from build123d import *

# Parameters (mm, degrees)
F4_W = 133.35
F4_H = 38.1
F0_W = 133.35
F0_H = 66.675
F6_T = -2.54


with BuildPart() as f5:
    # F4 (on face) → F5 section 0
    with BuildSketch(Plane(origin=(0, -59.055, 59.055), x_dir=(1, 0, 0), z_dir=(0, 0.7071067812, -0.7071067812))):
        with Locations((60.325, 0.0451280605)):
            Rectangle(F4_W, F4_H)
    # F0 (on Top) → F5 section 1
    with BuildSketch(Plane.XY):
        with Locations((60.325, 26.9875)):
            Rectangle(F0_W, F0_H)
    loft()

    # F6
    f6_openings = [f5.faces().sort_by_distance(p)[0] for p in [
        (60.325, 26.9875, 0),
        (60.325, -59.08691, 59.02309),
    ]]
    offset(amount=F6_T, openings=f6_openings)


solid = f5.part
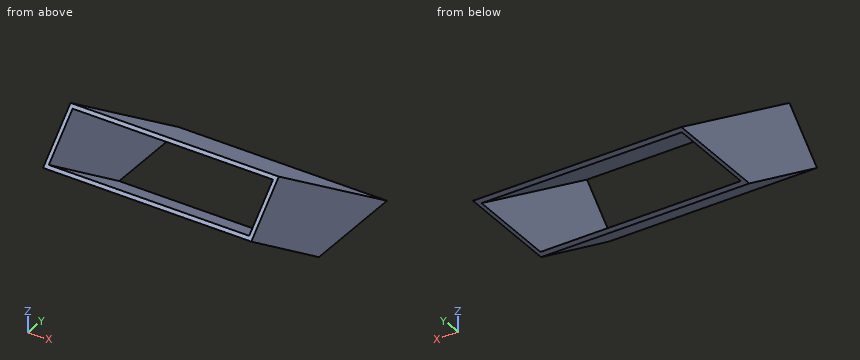
Can you work these out from the model? Positions are in its coordinate system, mm. Coordinates: 2 decimals unless noted, no trailing zeros. Write each loop counter-clockwise with the first axis right and the second up, starting at its lowest first coordinate (ties: lowest second). Pieces come first, ordered by that corner, then holes. Notation, with made-up numbers: (80.5, 5.25) - (123.5, 5.25) arc R29 ccw to (123.5, 38.25) - close; hole circle Ø8 at (-2, 45). An arc over 180 degrees is marked (long way). Return JSON: item names as keys, results as strings. Group by question number.
Item 1: If we section it at A-A (x = 74): Write out the boundary of the cut face in (y, z) (3 decimals), then the cut area to 3 significant figures.
Item 2: Please list where these lines run through material, in increasing order: probe 1 along X at (y, z) = (35, 8.5); probe 2 along Z at (x, y) = (76, -25); probe 3 along Y at (x, z) = (2.5, 45).
Item 3: I'm going to push flat-ended pins straight in: pin 1 Ø4 at (x, z) = (33, 18) entering from -Y; pin 2 Ø3 at (x, y) = (22.5, -18.5) entering from +Z; pin 3 Ø6 at (x, y) = (12, -50) entering from +Z; pin 4 Ø5 at (y, z) = (20, 33.5) entering from +X. Where does each tip first touch, or does it pass through?
Return value:
{
 "1": {"outline": "(-72.557, 45.553) - (-6.35, 0) - (-1.869, 0) - (-70.731, 47.379) - close; (-47.444, 70.666) - (55.827, 0) - (60.325, 0) - (-45.617, 72.493) - close", "area": "530 mm^2"},
 "2": {"probe 1": "x = -6.35 to -3.81, 124.46 to 127", "probe 2": "z = 12.83 to 15.91, 55.31 to 58.39", "probe 3": "y = -71.75 to -67.27, -9.94 to -5.44"},
 "3": {"pin 1": "stops at y = -35.42", "pin 2": "stops at z = 54.96", "pin 3": "stops at z = 71.11", "pin 4": "passes through"}
}
